Geometry: see drawing. Coordinates: mm, zero at the bounding-box minimum. A direction names the side the tool comes from. Round coordinates to 2 decimals unless told otherwise and drop trailing zeros. Loops run counter-clockwise (first coordinate to the right, second up) from the corner with the lowest first, then second, coordinate; pieces in that order, holes last.
(1) Cut plane D-D, the plane y = 13. Output: boundary loops of the cut face in (x, z), and give its area (3 significant figures).
(2) Line query: line 1 (Z direction, x = 31.5, y = 1) (1 decimal); line 2 (X direction, y = 14, z = 20); line 3 (Y direction, x = 7, z = 24). Output: solid intervals per line, ascending.
(3) Access query for the marked faces 4 and 5. Directions: +Z, -Z, +X, -X, +Y, -Y. A direction counts if a zero-diameter tool reaches every point of the face in a straight line with its end or side. Return the directions, or none.
(4) Cut plane A-A, the plane x = 20. Output: boundary loops of the cut face in (y, z).
(5) First-contact query: pin 1 Ø4 at (x, z) = (30.61, 9.39) entering from -Y; pin 2 Ø2 at (x, z) = (21.5, 20) entering from +Y; pin 3 Ø5 at (x, y) = (20, 13) entering from -Z; pin 4 Ø6 at (x, y) = (16, 13.5) entering from +Z (1 decimal). Flat tips, straight axial feed; report the tip coordinate or a pass-through.
(6) Cut plane B-B, the plane z = 20. Output: boundary loops of the cut face in (x, y), and give its area (3 significant figures).
(7) Cut plane C-C, the plane y = 16.5. Output: boundary loops of the cut face in (x, z), and give its area (3 significant figures).
(8) Draft query along Z for the marked faces 1, 2 and 3. Return one class per face: released by +Z, released by -Z, zero draft, split by the parting line, or undercut.
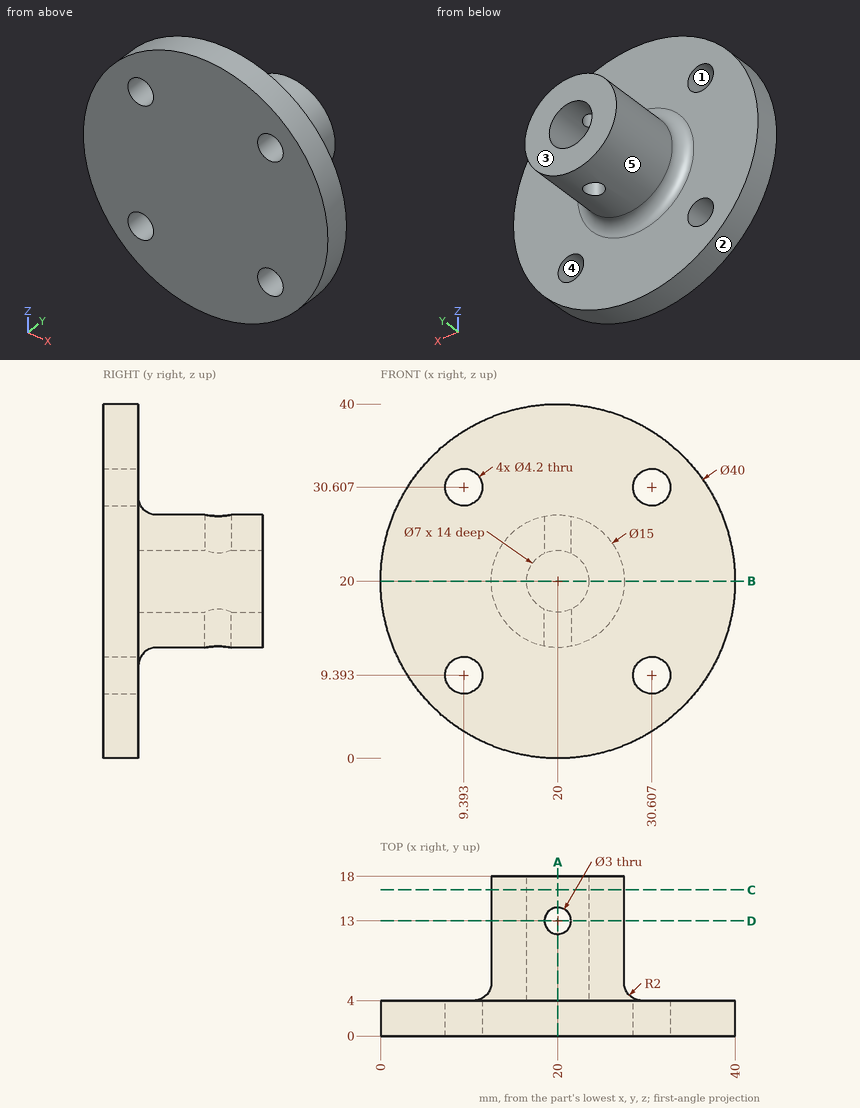
Reported:
1. outline: (18.5, 12.65) - (18.5, 16.84) arc R3.5 cw to (18.5, 23.16) - (18.5, 27.35) arc R7.5 ccw to start; (21.5, 12.65) arc R7.5 ccw to (21.5, 27.35) - (21.5, 23.16) arc R3.5 cw to (21.5, 16.84) - close
1. area: 114 mm2
2. line 1: z = 3.6 to 7.5, 11.3 to 28.7, 32.5 to 36.4
2. line 2: x = 12.5 to 16.5, 23.5 to 27.5
2. line 3: y = 0 to 4
3. face 4: +Y, -Y
3. face 5: +Y
4. outline: (0, 0) - (4, 0) - (4, 10.5) arc R2 cw to (6, 12.5) - (11.5, 12.5) - (11.5, 16.5) - (4, 16.5) - (4, 23.5) - (11.5, 23.5) - (11.5, 27.5) - (6, 27.5) arc R2 cw to (4, 29.5) - (4, 40) - (0, 40) - close; (14.5, 12.5) - (18, 12.5) - (18, 16.5) - (14.5, 16.5) - close; (14.5, 23.5) - (18, 23.5) - (18, 27.5) - (14.5, 27.5) - close
5. pin 1: passes through
5. pin 2: stops at y = 4
5. pin 3: stops at z = 12.5
5. pin 4: stops at z = 27.4
6. outline: (0, 0) - (40, 0) - (40, 4) - (29.5, 4) arc R2 cw to (27.5, 6) - (27.5, 18) - (23.5, 18) - (23.5, 4) - (16.5, 4) - (16.5, 18) - (12.5, 18) - (12.5, 6) arc R2 cw to (10.5, 4) - (0, 4) - close
6. area: 274 mm2
7. outline: circle Ø15 at (20, 20); hole circle Ø7 at (20, 20)
7. area: 138 mm2
8. face 1: undercut
8. face 2: split by the parting line
8. face 3: zero draft
